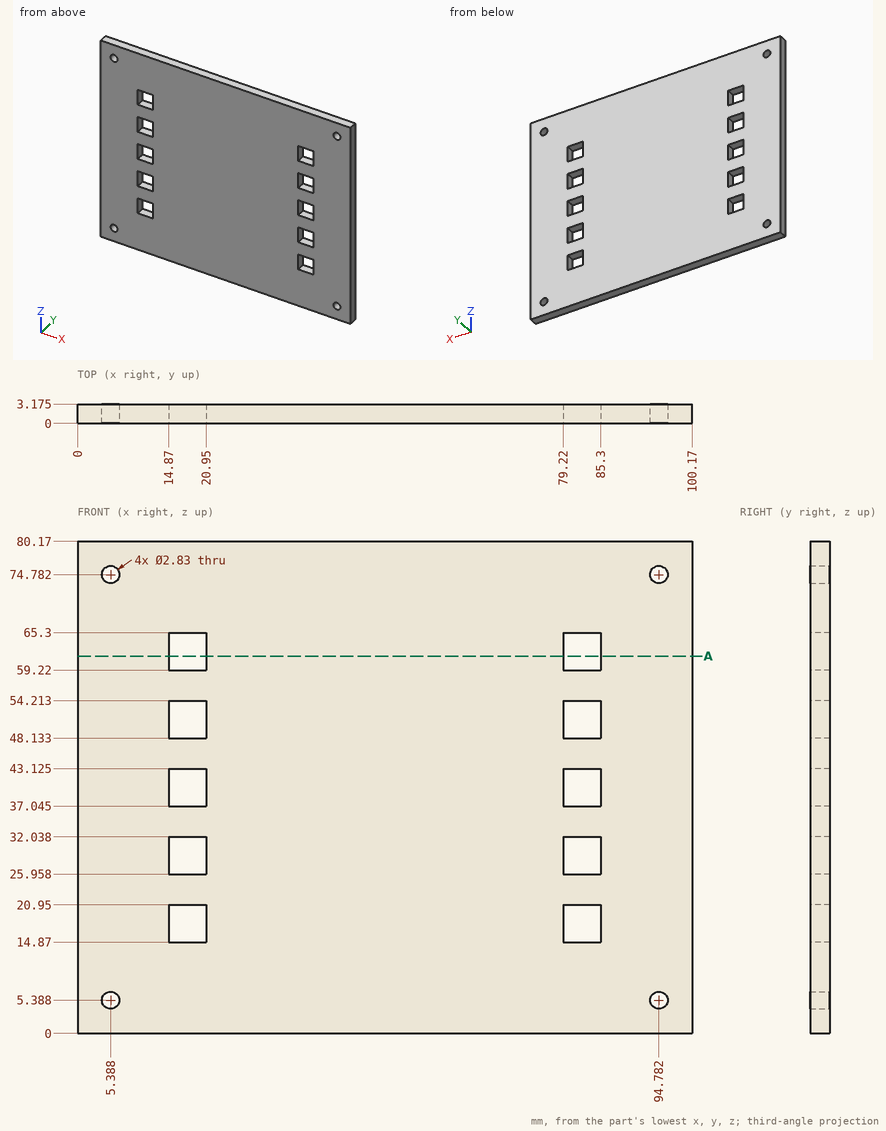
Can you work these out from the drawing? Everything is in mm from the part's minimum corner. Round coordinates to 2 decimals unless told otherwise and drop trailing zeros. Put each result on its own line as item: value.
Q1. I want a section at A-A on z = 61.5. Give the number of separate pieces and of enclosed holes in the cut face.
Checks:
separate pieces: 3
enclosed holes: 0
Q2. For pin 1 Ø2.5 at (x, z) = (94.78, 5.39) entering from -Y, with a flat end and sliding along its axis, tell me the tip position at first contact or that it passes through.
Checks:
pin 1: through
Q3. Please list where these lines run through material, in increasing order: line 1 (X direction, y = 1.5, z = 49.5); line 2 (X direction, y = 1.75, z = 75.5). Write a range as from..to.
Checks:
line 1: 0..14.87, 20.95..79.22, 85.3..100.17
line 2: 0..4.17, 6.61..93.56, 96..100.17
